from build123d import *

# Parameters (mm, degrees)
CUT_EXTRUDE1_DEPTH = 1
CHAMFER1_SIZE      = 0.3


with BuildPart() as part:
    # Sketch1 → Revolve1 (revolve)
    with BuildSketch(Plane(origin=(0, 0, 0), x_dir=(1, 0, 0), z_dir=(0, 1, 0))):
        with BuildLine():
            Line((3, 0), (3, -0.5))
            Line((3, -0.5), (1.5, -2))
            Line((1.5, -2), (1.5, -3.985079935))
            Line((1.5, -3.985079935), (0, -3.985079935))
            Line((0, -3.985079935), (0, 0.619607068))
            ThreePointArc((0, 0.619607068), (1.531658653, 0.463087711), (3, 0))
        make_face()
    revolve(axis=Axis((0, 0, 3.985079935), (0, 0, -1)))

    # Sketch2 → Cut-Extrude1 (cut)
    with BuildSketch(Plane.XY.offset(-0.619607068)):
        Polygon((1.5, 0), (0.75, 1.299038106), (-0.75, 1.299038106), (-1.5, 0), (-0.75, -1.299038106), (0.75, -1.299038106), align=None)
    extrude(amount=CUT_EXTRUDE1_DEPTH, mode=Mode.SUBTRACT)

    # Chamfer1
    chamfer1_edges = [part.edges().sort_by_distance(p)[0] for p in [
        (1.125, -0.649519053, 0.380392932),
        (1.125, 0.649519053, 0.380392932),
        (0, 1.299038106, 0.380392932),
        (-1.125, 0.649519053, 0.380392932),
        (-1.125, -0.649519053, 0.380392932),
        (0, -1.299038106, 0.380392932),
    ]]
    chamfer(chamfer1_edges, length=CHAMFER1_SIZE)


solid = part.part
CAD build for the part. Positions are in the model's coordinates, mm. A direction names the side the tool comes from. Coordinates: 2 decimals unless noted, no trailing zeros. Loops run counter-clockwise (first coordinate to the right, second up) from the corner with the lowest first, then second, coordinate; pieces in that order, holes last. Notation, with made-up numbers: (30.5, 58.5) - (87.5, 58.5) arc R27 ccw to (87.5, 92.5) - close; hole circle Ø6 at (17.5, -7). An arc over 180 degrees is marked (long way). Write item = value, one per line. Start each with the question number.
Q1. Cut at B-B, the plane z = 0.6. List the corners of the cut face in (x, y).
Q2. Cut at A-A, the plane x = 0. List the corners of the cut face in (y, z), then the cut area to 3 significant figures.
Q3. Cut at C-C, the plane z = 1.45. List the corners of the cut face in (x, y).
Q4. Which spindle directions (+Z, -Z, +X, -X, +Y, -Y) get a long thin tool onto all of the face, cutting with end or side? Do faces 1 (the flat face through (0, 0, 0.38)), 2 (the cylindrical face through (-1.5, -0.07, 3.01)). Say none if no direction does.
Q5. Flat gauge pins, fed straight in: pin 1 Ø1.5 at (x, z) = (2, 3) entering from -Y; pin 2 Ø2 at (x, z) = (2.5, 0.5) entering from +Y; pin 3 Ø1 at (x, z) = (-1.5, 2) entering from +Y. Where does each tip first touch, or does it go through?
Q6. Pull direction X, two halves, no side cores. Call faces 3 (the flat face through (0.999, 0.564, 0.232)), 4 (the flat face through (-0.99, 0.58, 0.23)), 5 (the cylindrical face through (-3, -0.1, 0.3)), 6 (the flat face through (0, 0, 3.985)): pulls with the +X half, pulls with the -X half, needs draft (parallel to the pull), parting line crosses it, or undercut.
Q7. Drill centre lines: L1, parallel to Z at x = -0.3, y = -0.25; L2, parallel to Y at x = -1.3, z = 2.9; L3, parallel to X at y = -0.8, z = 2.5. Where is each one in solid material? Low to high.
Computed:
q1.outline = circle Ø5.8 at (0, 0)
q2.outline = (-3, 0) arc R7.57 ccw to (-1.3, -0.51) - (-1.3, 0.08) - (-1, 0.38) - (1, 0.38) - (1.3, 0.08) - (1.3, -0.51) arc R7.57 ccw to (3, 0) - (3, 0.5) - (1.5, 2) - (1.5, 3.99) - (-1.5, 3.99) - (-1.5, 2) - (-3, 0.5) - close
q2.area = 15.8 mm²
q3.outline = circle Ø4.1 at (0, 0)
q4.face_1 = -Z
q4.face_2 = +Z
q5.pin_1 = -0.83
q5.pin_2 = 2.6
q5.pin_3 = 1.48
q6.face_3 = undercut
q6.face_4 = undercut
q6.face_5 = parting line crosses it
q6.face_6 = needs draft
q7.L1 = 0.38 to 3.99
q7.L2 = -0.75 to 0.75
q7.L3 = -1.27 to 1.27
